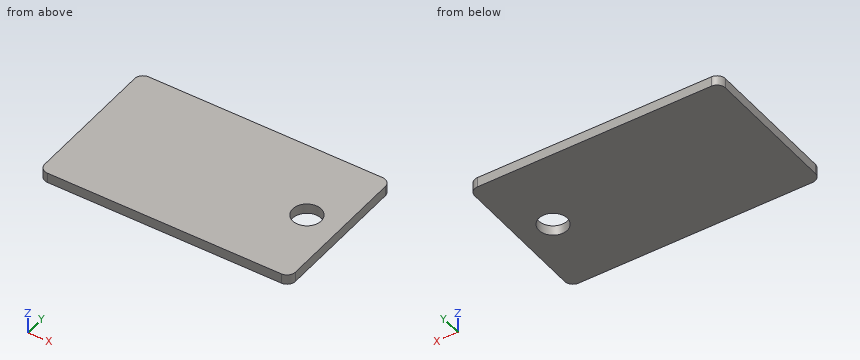
Autodesk Inventor part; units mm, degrees
ref_plane "YZ Plane" through (0, 0, 0) normal (1, 0, 0) x (0, 1, 0)
ref_plane "XZ Plane" through (0, 0, 0) normal (0, 1, 0) x (-1, 0, 0)
ref_plane "XY Plane" through (0, 0, 0) normal (0, 0, 1) x (1, 0, 0)
sketch "Sketch1" plane through (0, 0, 0) normal (0, 0, 1) x (1, 0, 0)
  line L0 (-75, -45) -> (75, -45)
  line L1 (75, -45) -> (75, 45)
  line L2 (75, 45) -> (-75, 45)
  line L3 (-75, 45) -> (-75, -45)
  line L4 (-75, -45) -> (75, 45) construction
  line L5 (75, -45) -> (-75, 45) construction
  circle A0 centre (55, -25) radius 8.5
  circle A1 centre (55, 25) radius 8.5
  line L6 (0, 0) -> (75, 0) construction
  circle A2 centre (55, 0) radius 8.5
  dimension "d0" = 150
  dimension "d1" = 90
  dimension "d23" = 17
  dimension "d25" = 20
  dimension "d26" = 20
extrude "Plate1" add sketch "Sketch1" along normal blind 6 contours L3 L2 L1 L0 | A0 | A1
fillet "Corner Round2" radius 5 4 edges at (-75, 45, 3) (-75, -45, 3) (75, -45, 3) (75, 45, 3)
equation "\"d26\" = d25"
equation "\"d2\" = Thickness"
equation "\"BendReliefWidth\" = Thickness"
equation "\"BendReliefDepth\" = 0.5 * Thickness"
equation "\"CornerReliefSize\" = 4 * Thickness"
equation "\"MinimumRemnant\" = 2 * Thickness"
equation "\"TransitionRadius\" = BendRadius"
equation "\"JacobiRadiusSize\" = BendRadius"
equation "\"GapSize\" = Thickness"
properties part number "PRS 1200-94 leg floor plate" material "Stainless Steel"
Verification items for the finished model (mm, model axes). Coordinates: 2 decimals unless noted, no trailing zeros. Loops run counter-clockwise (first coordinate to the right, second up) from the corner with the lowest first, then second, coordinate; pieces in that order, holes last. Notation, with made-up numbers: (3.5, 3) - (11.5, 3) arc R37 ccw to (11.5, 40) - close; hole circle Ø2 at (47.25, 19). An arc over 180 degrees is marked (long way). Return JSON: item names as keys, results as strings.
1. Section check B-B, the plane x = 55. Record the boundary of the cut face in (y, z).
Established:
{"outline": "(-45, 0) - (-8.5, 0) - (-8.5, 6) - (-45, 6) - close; (8.5, 0) - (45, 0) - (45, 6) - (8.5, 6) - close"}
2. Section check A-A, the plane y = 0. Record the boundary of the cut face in (x, z).
Established:
{"outline": "(-75, 0) - (46.5, 0) - (46.5, 6) - (-75, 6) - close; (63.5, 0) - (75, 0) - (75, 6) - (63.5, 6) - close"}
3. Thickness scan on L1, parallel to Y at x = 55, z = 2.1; L2, parallel to X at y = -2, z = 4.95; L3, parallel to X at y = -3, z = 4. Record the ranges inside material, lowest first.
Established:
{"L1": "y = -45 to -8.5, 8.5 to 45", "L2": "x = -75 to 46.74, 63.26 to 75", "L3": "x = -75 to 47.05, 62.95 to 75"}
4. Section check C-C, the plane z = 3.65. Record the boundary of the cut face in (x, y).
Established:
{"outline": "(-75, -40) arc R5 ccw to (-70, -45) - (70, -45) arc R5 ccw to (75, -40) - (75, 40) arc R5 ccw to (70, 45) - (-70, 45) arc R5 ccw to (-75, 40) - close; hole circle Ø17 at (55, 0)"}
